```python
from build123d import *

# Parameters (mm, degrees)
F0_W      = 43.18
F0_H      = 25.4
F1_DEPTH  = 25.4
F2_W      = 17.78
F2_H      = 25.4
F3_DEPTH  = 25.4
F4_W      = 25.4
F4_H      = 25.4
F5_DEPTH  = 50.8
F6_W      = 22.86
F6_H      = 25.4
F7_DEPTH  = 25.4
F8_W      = 25.4
F8_H      = 25.4
F9_DEPTH  = 58.42
F10_W     = 17.78
F10_H     = 25.4
F11_DEPTH = 25.4
F12_W     = 25.4
F12_H     = 17.78
F13_DEPTH = 25.4


with BuildPart() as f1:
    # F0 (on Right) → F1 (new body)
    with BuildSketch(Plane.YZ):
        with Locations((36.3900898956, -36.7231099647)):
            Rectangle(F0_W, F0_H)
    extrude(amount=F1_DEPTH)

    # F2 (on face) → F3 (join)
    with BuildSketch(Plane(origin=(0, 0, 0), x_dir=(0, -1, 0), z_dir=(-1, 0, 0))):
        with Locations((-23.6900898956, -36.7231099647)):
            Rectangle(F2_W, F2_H)
    extrude(amount=F3_DEPTH)

    # F4 (on face) → F5 (join)
    with BuildSketch(Plane.XZ.offset(-14.8000898956)):
        with Locations((-12.7, -36.7231099647)):
            Rectangle(F4_W, F4_H)
    extrude(amount=F5_DEPTH)

    # F6 (on face) → F7 (join)
    with BuildSketch(Plane(origin=(-25.4, 0, 0), x_dir=(0, -1, 0), z_dir=(-1, 0, 0))):
        with Locations((24.5699101044, -36.7231099647)):
            Rectangle(F6_W, F6_H)
    extrude(amount=F7_DEPTH)

    # F8 (on face) → F9 (join)
    with BuildSketch(Plane.XZ.offset(35.9999101044)):
        with Locations((-38.1, -36.7231099647)):
            Rectangle(F8_W, F8_H)
    extrude(amount=F9_DEPTH)

    # F10 (on face) → F11 (join)
    with BuildSketch(Plane.YZ.offset(-25.4)):
        with Locations((-85.5299101044, -36.7231099647)):
            Rectangle(F10_W, F10_H)
    extrude(amount=F11_DEPTH)

    # F12 (on face) → F13 (join)
    with BuildSketch(Plane.XY.offset(-24.0231099647)):
        with Locations((-12.7, -85.5299101044)):
            Rectangle(F12_W, F12_H)
    extrude(amount=F13_DEPTH)


solid = f1.part
```
Input: part model. Units: mm. Frame: model coordinates. A direction names the side the tool comes from. Give positions to 0.01 mm unless a question says otherwise; leave off trailing zeros. Order: outer loops, then holes, each group sorted by start corner. A loop starts at its lowest first (then second) coordinate and runs counter-clockwise, first axis right, second up.
1. Reachability of faces 4 (the flat face through (0, -86, -24)), 5 (the flat face through (-25.4, -86, -12)), 6 (the flat face through (-13, 32.58, -37)), 7 (the flat face through (-13, -36, -37)) from +Z, -Z, +X, -X, +Y, -Y: full face, straight path, thin tool, end or side. Return the list, or none.
Derived:
face 4: +Z, -Z, +X, -Y
face 5: +Z, -X, +Y, -Y
face 6: +Z, -Z, -X, +Y
face 7: +Z, -Z, +X
2. Section D-D on x = -34. Return the cut outline in (y, z).
Derived:
outline: (-94.42, -49.42) - (-13.14, -49.42) - (-13.14, -24.02) - (-94.42, -24.02) - close
3. Section A-A on x = -7.5. Return the cut outline in (y, z), and give its area (3 significant figures).
Derived:
outline: (-94.42, -49.42) - (-76.64, -49.42) - (-76.64, 1.38) - (-94.42, 1.38) - close; (-36, -49.42) - (32.58, -49.42) - (32.58, -24.02) - (-36, -24.02) - close
area: 2,650 mm2
4. Mould query, pull axis Y, two halves, no side actions, for faces 1 (the flat face through (0, -10, -37)), 2 (the flat face through (-13, -76.64, -24)), 3 (the flat face through (-20, -94.42, -30)). Classes: released by +Y, released by -Y, zero draft, split by the parting line, or undercut.
Derived:
face 1: zero draft
face 2: undercut
face 3: released by -Y
5. Material intervals for L1, parallel to Z at x = 19, y = 21.5; L2, parallel to X at y = 19, z = -30; L3, parallel to Y at x = -3.5, z = -22, sorted ascending.
Derived:
L1: z = -49.42 to -24.02
L2: x = -25.4 to 25.4
L3: y = -94.42 to -76.64
6. Pin query (flat end, axial travel): pin 1 (12.5 mm diameter, centred on x = 11.5, z = -40.5, fed in from -Y); pin 2 (12.5 mm diameter, centred on x = -8.5, z = -36.5, fed in from +Y); pin 3 (9 mm diameter, centred on y = -83.5, z = -16.5, fed in from -X); pin 4 (12 mm diameter, centred on x = 8, y = 0, fed in from -Z). Return the tip coordinate at first contact, or that it passes through.
Derived:
pin 1: stops at y = 14.8
pin 2: stops at y = 32.58
pin 3: stops at x = -25.4
pin 4: passes through
7. Section B-B on z = -44. Return the cut outline in (x, y).
Derived:
outline: (-50.8, -94.42) - (0, -94.42) - (0, -76.64) - (-25.4, -76.64) - (-25.4, -36) - (0, -36) - (0, 14.8) - (25.4, 14.8) - (25.4, 57.98) - (0, 57.98) - (0, 32.58) - (-25.4, 32.58) - (-25.4, -13.14) - (-50.8, -13.14) - close
8. Section C-C on y = -80. Return the cut outline in (x, z).
Derived:
outline: (-50.8, -49.42) - (0, -49.42) - (0, 1.38) - (-25.4, 1.38) - (-25.4, -24.02) - (-50.8, -24.02) - close
